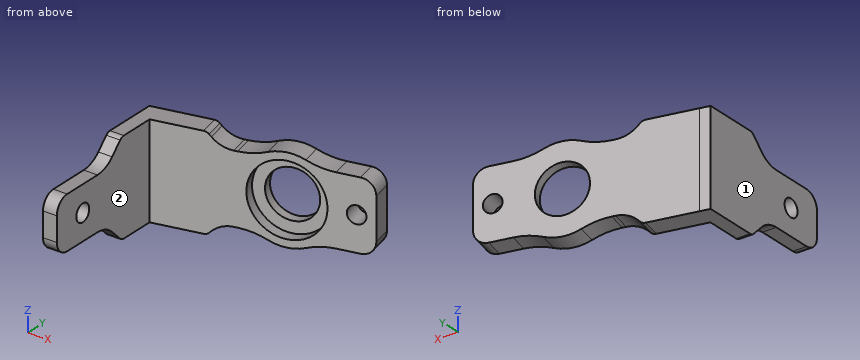
```python
from build123d import *

# Parameters (mm, degrees)
BOSS_EXTRUDE1_DEPTH     = 3
BOSS_EXTRUDE2_DEPTH     = 2
CUT_EXTRUDE1_DEPTH      = 7.75
CUT_EXTRUDE1_DEPTH_BACK = 7.75
SKETCH5_R               = 1.25
CUT_EXTRUDE2_DEPTH      = 31.070572477
SKETCH6_R               = 1.25
CUT_EXTRUDE3_DEPTH      = 27.558218913
SKETCH7_R               = 3.5
CUT_EXTRUDE4_DEPTH      = 27.558218913
SKETCH10_R              = 6.25
SKETCH10_R_2            = 3.5
BOSS_EXTRUDE3_DEPTH     = 3
SKETCH8_R               = 5.15
CUT_EXTRUDE5_DEPTH      = 1.6
FILLET1_R               = 10


with BuildPart() as part:
    # Sketch2 → Boss-Extrude1 (new body)
    with BuildSketch(Plane(origin=(-8.299779748, 37.326456989, 0), x_dir=(0.976159298, 0.21705535, 0), z_dir=(-0.21705535, 0.976159298, 0))):
        with BuildLine():
            Line((-4.14298056, 6.75), (-8.912705405, 6.75))
            Line((-8.912705405, 6.75), (-8.912705405, -6.75))
            Line((-8.912705405, -6.75), (-4.14298056, -6.75))
            Line((-4.14298056, -6.75), (-3.64298056, -6.75))
            Line((-3.64298056, -6.75), (-2.057194122, -6.75))
            ThreePointArc((-2.057194122, -6.75), (-1.67451069, -6.673879533), (-1.350087341, -6.457106781))
            Line((-1.350087341, -6.457106781), (-1.064553435, -6.171572875))
            ThreePointArc((-1.064553435, -6.171572875), (0.23313996, -5.30448187), (1.76387369, -5))
            Line((1.76387369, -5), (14.343433612, -5))
            Line((14.343433612, -5), (14.843433612, -5))
            Line((14.843433612, -5), (17.843433612, -5))
            ThreePointArc((17.843433612, -5), (19.257647174, -4.414213562), (19.843433612, -3))
            Line((19.843433612, -3), (19.843433612, 3))
            ThreePointArc((19.843433612, 3), (19.257647174, 4.414213562), (17.843433612, 5))
            Line((17.843433612, 5), (14.843433612, 5))
            Line((14.843433612, 5), (14.343433612, 5))
            Line((14.343433612, 5), (1.76387369, 5))
            ThreePointArc((1.76387369, 5), (0.23313996, 5.30448187), (-1.064553435, 6.171572875))
            Line((-1.064553435, 6.171572875), (-1.350087341, 6.457106781))
            ThreePointArc((-1.350087341, 6.457106781), (-1.67451069, 6.673879533), (-2.057194122, 6.75))
            Line((-2.057194122, 6.75), (-3.64298056, 6.75))
            Line((-3.64298056, 6.75), (-4.14298056, 6.75))
        make_face()
    extrude(amount=BOSS_EXTRUDE1_DEPTH)

    # Sketch3 → Boss-Extrude2 (add)
    with BuildSketch(Plane.ZY.offset(17)):
        with BuildLine():
            Line((-6.75, 35.391906601), (-6.75, 38.320384496))
            Line((-6.75, 38.320384496), (6.75, 38.320384496))
            Line((6.75, 38.320384496), (6.75, 35.391906601))
            Line((6.75, 35.391906601), (6.75, 30.414213562))
            ThreePointArc((6.75, 30.414213562), (6.673879533, 30.03153013), (6.457106781, 29.707106781))
            Line((6.457106781, 29.707106781), (4.921572875, 28.171572875))
            ThreePointArc((4.921572875, 28.171572875), (4.05448187, 26.87387948), (3.75, 25.343145751))
            Line((3.75, 25.343145751), (3.75, 20.3))
            Line((3.75, 20.3), (3.75, 19.8))
            Line((3.75, 19.8), (3.75, 19.5))
            ThreePointArc((3.75, 19.5), (3.164213562, 18.085786438), (1.75, 17.5))
            Line((1.75, 17.5), (-1.75, 17.5))
            ThreePointArc((-1.75, 17.5), (-3.164213562, 18.085786438), (-3.75, 19.5))
            Line((-3.75, 19.5), (-3.75, 19.8))
            Line((-3.75, 19.8), (-3.75, 20.3))
            Line((-3.75, 20.3), (-3.75, 25.343145751))
            ThreePointArc((-3.75, 25.343145751), (-4.05448187, 26.87387948), (-4.921572875, 28.171572875))
            Line((-4.921572875, 28.171572875), (-6.457106781, 29.707106781))
            ThreePointArc((-6.457106781, 29.707106781), (-6.673879533, 30.03153013), (-6.75, 30.414213562))
            Line((-6.75, 30.414213562), (-6.75, 35.391906601))
        make_face()
    extrude(amount=BOSS_EXTRUDE2_DEPTH)

    # Sketch4 → Cut-Extrude1 (cut, two sides)
    with BuildSketch(Plane.XY) as cut_extrude1_sk:
        Polygon((-17.651166049, 38.320384496), (-19, 38.02046252), (-19, 38.320384496), align=None)
    extrude(amount=CUT_EXTRUDE1_DEPTH, mode=Mode.SUBTRACT)
    extrude(cut_extrude1_sk.sketch, amount=-CUT_EXTRUDE1_DEPTH_BACK, mode=Mode.SUBTRACT)

    # Sketch5 → Cut-Extrude2 (cut, through all)
    with BuildSketch(Plane.ZY.offset(19)):
        with Locations((0, 22.5)):
            Circle(SKETCH5_R)
    extrude(amount=-CUT_EXTRUDE2_DEPTH, mode=Mode.SUBTRACT)

    # Sketch6 → Cut-Extrude3 (cut, through all)
    with BuildSketch(Plane(origin=(-8.950945797, 40.254934884, 0), x_dir=(0.976159298, 0.21705535, 0), z_dir=(-0.21705535, 0.976159298, 0))):
        with Locations((17.343433612, 0)):
            Circle(SKETCH6_R)
    extrude(amount=-CUT_EXTRUDE3_DEPTH, mode=Mode.SUBTRACT)

    # Sketch7 → Cut-Extrude4 (cut, through all)
    with BuildSketch(Plane(origin=(-8.950945797, 40.254934884, 0), x_dir=(0.976159298, 0.21705535, 0), z_dir=(-0.21705535, 0.976159298, 0))):
        with Locations((8.502484958, 0)):
            Circle(SKETCH7_R)
    extrude(amount=-CUT_EXTRUDE4_DEPTH, mode=Mode.SUBTRACT)

    # Sketch10 → Boss-Extrude3 (add)
    with BuildSketch(Plane(origin=(-8.950945797, 40.254934884, 0), x_dir=(0.976159298, 0.21705535, 0), z_dir=(-0.21705535, 0.976159298, 0))):
        with Locations((8.502484958, 0)):
            Circle(SKETCH10_R)
        with Locations((8.502484958, 0)):
            Circle(SKETCH10_R_2, mode=Mode.SUBTRACT)
    extrude(amount=-BOSS_EXTRUDE3_DEPTH)

    # Sketch8 → Cut-Extrude5 (cut)
    with BuildSketch(Plane(origin=(-8.299779748, 37.326456989, 0), x_dir=(0.976159298, 0.21705535, 0), z_dir=(0.21705535, -0.976159298, 0))):
        with Locations((8.502484958, 0)):
            Circle(SKETCH8_R)
    extrude(amount=-CUT_EXTRUDE5_DEPTH, mode=Mode.SUBTRACT)

    # Fillet1
    fillet1_edges = [part.edges().sort_by_distance(p)[0] for p in [
        (-3.986180392, 39.822248221, 5),
        (-3.986180392, 39.822248221, -5),
        (3.335014343, 41.450163343, 5),
        (3.335014343, 41.450163343, -5),
    ]]
    fillet(fillet1_edges, radius=FILLET1_R)


solid = part.part
```
Model file for the job. Use its own axes, mm. Face numbers are marked on the shaded views. A direction names the side the tool comes from. Give positions to 0.01 mm unless a question says otherwise; leave off trailing zeros. Order: outer loops, then holes, each group sorted by start corner. A loop starts at its lowest first (then second) coordinate and runs counter-clockwise, first axis right, second up.
1) Saw through at C-C, the plane y = 36.5. Write the cut outline in (x, z).
2) Wall check: probe 1 along X at (y, z) = (34, 2.5); probe 2 along Z at (x, y) = (2, 40.25); probe 3 along Y at (x, z) = (-18.3, 0). Give the ranges that are in metal, low to high.
3) Saw through at A-A, the plane y = 22.5. Write the cut outline in (x, z), then the cut area to 3 significant figures.
4) Saw through at B-B, the plane z = -0.5. Write the cut outline in (x, y), then the cut area to 3 significant figures.
5) Saw through at D-D, the plane x = -13.5. Write the cut outline in (y, z), then the cut area to 3 significant figures.
6) 3-axis set-ups, long thin cutter, end or side, ignore diameter. For the marked faces 1 and 2: which of +Z, -Z, +X, -X, +Y, -Y reach the whole face in a straight line?
7) Pin check, flat tips, straight feed: pin 1 (5 mm diameter, centred on x = -7, z = -0.5, fed in from -Y); pin 2 (3 mm diameter, centred on y = 27, z = -4.5, fed in from +X); pin 3 (0.6 mm diameter, centred on x = -6.5, y = 39.5, fed in from +Z). Stop position of each tip, or through.
Computed:
1. outline: (-19, -6.75) - (-12.02, -6.75) - (-12.02, 6.75) - (-19, 6.75) - close
2. probe 1: x = -19 to -17
2. probe 2: z = -5.86 to -4.66, 4.66 to 5.86
2. probe 3: y = 17.5 to 21.25, 23.75 to 38.18
3. outline: (-19, -3.75) - (-17, -3.75) - (-17, -1.25) - (-19, -1.25) - close; (-19, 1.25) - (-17, 1.25) - (-17, 3.75) - (-19, 3.75) - close
3. area: 10.0 mm2
4. outline: (-19, 17.5) - (-17, 17.5) - (-17, 21.35) - (-19, 21.35) - close; (-19, 23.65) - (-17, 23.65) - (-17, 35.39) - (-5, 38.06) - (-5.35, 39.62) - (-3.73, 39.98) - (-4.03, 41.35) - (-19, 38.02) - close; (2.73, 42.85) - (3.03, 41.49) - (4.66, 41.85) - (5, 40.28) - (7.51, 40.84) - (6.86, 43.77) - close; (9.1, 44.27) - (9.75, 41.34) - (11.07, 41.63) - (10.42, 44.56) - close
4. area: 89.2 mm2
5. outline: (36.17, -6.75) - (39.24, -6.75) - (39.24, 6.75) - (36.17, 6.75) - close
5. area: 41.5 mm2
6. face 1: +Z, -Z, -X, +Y, -Y
6. face 2: +Z, -Z, +X, -Y
7. pin 1: stops at y = 37.06
7. pin 2: stops at x = -17
7. pin 3: stops at z = 5
